Autodesk Inventor part; units mm, degrees
ref_plane "YZ Plane" through (0, 0, 0) normal (1, 0, 0) x (0, 1, 0)
ref_plane "XZ Plane" through (0, 0, 0) normal (0, 1, 0) x (-1, 0, 0)
ref_plane "XY Plane" through (0, 0, 0) normal (0, 0, 1) x (1, 0, 0)
sketch "Sketch1" plane through (0, 0, 0) normal (0, 1, 0) x (-1, 0, 0)
  line L0 (0, 0) -> (349.25, 0)
  line L1 (349.25, 0) -> (349.25, -400.05)
  line L2 (349.25, -400.05) -> (0, -400.05)
  line L3 (0, -400.05) -> (0, 0)
  dimension "d0" = 400.05
  dimension "d1" = 349.25
extrude "Extrusion1" add sketch "Sketch1" along normal blind 352.425
sketch "Sketch2" plane through (0, 0, 0) normal (1, 0, 0) x (0, 0, -1)
  line L0 (30.1625, 339.725) -> (369.8875, 339.725)
  line L1 (369.8875, 339.725) -> (369.8875, 12.7)
  line L2 (369.8875, 12.7) -> (30.1625, 12.7)
  line L3 (30.1625, 12.7) -> (30.1625, 339.725)
  line L4 (0, 0) -> (400.05, 0)
  line L5 (0, 352.425) -> (400.05, 352.425)
  line L6 (0, 0) -> (0, 352.425)
  line L7 (400.05, 0) -> (400.05, 352.425)
  dimension "d4" = 12.7
  dimension "d5" = 12.7
  dimension "d6" = 339.725
  dimension "d7" = 30.1625
  dimension "d8" = 30.1625
extrude "Extrusion2" cut sketch "Sketch2" against normal blind 333.375 contours L0 L1 L2 L3
sketch "Sketch3" plane through (0, 352.425, 0) normal (0, 1, 0) x (1, 0, 0)
  line L0 (0, 400.05) -> (-349.25, 400.05)
  line L1 (-349.25, 400.05) -> (-349.25, 0)
  line L2 (-349.25, 0) -> (0, 0)
  line L3 (0, 0) -> (0, 400.05)
extrude "Extrusion3" add sketch "Sketch3" along normal blind 174.625
sketch "Sketch4" plane through (0, 0, 0) normal (1, 0, 0) x (0, 0, -1)
  line L0 (369.8875, 339.725) -> (369.8875, 12.7)
  line L1 (369.8875, 12.7) -> (30.1625, 12.7)
  line L2 (30.1625, 12.7) -> (30.1625, 339.725)
  line L3 (30.1625, 339.725) -> (369.8875, 339.725)
  line L4 (0, 0) -> (400.05, 0)
  line L5 (400.05, 0) -> (400.05, 527.05)
  line L6 (0, 527.05) -> (400.05, 527.05)
  line L7 (0, 0) -> (0, 527.05)
  line L8 (30.1625, 501.65) -> (369.8875, 501.65)
  line L9 (369.8875, 501.65) -> (369.8875, 352.425)
  line L10 (369.8875, 352.425) -> (30.1625, 352.425)
  line L11 (30.1625, 352.425) -> (30.1625, 501.65)
  point P0 (200.025, 501.65)
  dimension "d13" = 12.7
  dimension "d14" = 25.4
extrude "Extrusion4" cut sketch "Sketch4" against normal blind 333.375 contours L8 L9 L10 L11
sketch "Sketch5" plane through (0, 527.05, 0) normal (0, 1, 0) x (1, 0, 0)
  line L0 (-349.25, 400.05) -> (-349.25, 0)
  line L1 (-349.25, 0) -> (0, 0)
  line L2 (0, 0) -> (0, 400.05)
  line L3 (0, 400.05) -> (-349.25, 400.05)
  circle A0 centre (-169.8625, 200.025) radius 63.5
  line L4 (-106.3625, 200.025) -> (0, 200.025) construction
  dimension "d17" = 127
  dimension "d20" = 106.3625
extrude "Extrusion5" cut sketch "Sketch5" against normal blind 193.675 contours A0
sketch "Sketch6" plane through (0, 527.05, 0) normal (0, 1, 0) x (1, 0, 0)
  line L0 (-312.7375, 123.825) -> (-265.1125, 123.825)
  line L1 (-265.1125, 123.825) -> (-265.1125, 276.225)
  line L2 (-265.1125, 276.225) -> (-312.7375, 276.225)
  line L3 (-312.7375, 276.225) -> (-312.7375, 123.825)
  line L4 (-349.25, 400.05) -> (-349.25, 0)
  line L5 (-349.25, 0) -> (0, 0)
  line L6 (0, 400.05) -> (-349.25, 400.05)
  line L7 (0, 0) -> (0, 400.05)
  circle A0 centre (-169.8625, 200.025) radius 63.5
  line L8 (-233.3625, 200.025) -> (-265.1125, 200.025)
  dimension "d23" = 152.4
  dimension "d24" = 47.625
  dimension "d26" = 123.825
  dimension "d27" = 123.825
  dimension "d32" = 265.1125
extrude "Extrusion6" add sketch "Sketch6" along normal blind 3.175 and the other way blind 38.1 contours L3 L2 L1 L0
properties part number "Table"
Can you work these out from the model? Positions are in its coordinate system, mm. A direction names the side the tool comes from. Give positions to 0.01 mm unless a question says otherwise; leave off trailing zeros. Loops run counter-clockwise (first coordinate to the right, second up) from the corner with the lowest first, then second, coordinate; pieces in that order, holes last. Notation, with made-up numbers: M 83.25,-11 L 129.25,-11 A11 ccw 129.25,1 Z; hole C 38,41.25 d11. An arc over 180 degrees is marked long. One line per item, written item: value. Start each with the question number.
1) Thinking about a two-plate mould opening in Z: for faces 4 (the face through (-164, 174, -30.162)), 5 (the face through (-289, 530.225, -201)), 6 (the face through (-177, 260, 0)), which applies, +Z half, -Z half, draft (parallel to the pull), parting line (faces both ways), or undercut?
2) If we section it at B-B, the plane x = -60: Give the number of separate pieces and of enclosed holes in the cut face, and give its area (3 significant figures).
3) I'm going to push flat-ended pins straight in: pin 1 (1.6 mm diameter, centred on y = 528, z = -227.5, fed in from -X); pin 2 (12 mm diameter, centred on x = -40.5, z = -179.5, fed in from +Y); pin 3 (2 mm diameter, centred on y = 312.5, z = -297, fed in from +X) (3 decimals); pin 4 (10 mm diameter, centred on x = -168.5, y = 176, fed in from +Z). Where does each tip first touch, or does it pass through?
4) If we section it at C-C, the plane z = -111.5: Write out the boundary of the cut face in (x, y) (3 decimals), and give its area (3 significant figures).
5) If I drill on line 1 (Y direction, x = -36, z = -362) (3 decimals); line 2 (Z direction, x = -209.5, y = 407); line 3 (X direction, y = 259, z = -323.5) (3 decimals), over which ranges is the centre line in solid material (lowest first)? Write a range as [from, to].
6) On a 3-axis mill with a long thin cutter (end or side, diameter ignored), from which of +Z, -Z, +X, -X, +Y, -Y can I reach the whole of each face in a straight line? I mean faces 1 (the face through (-312.738, 495, -201)), 2 (the face through (-289, 488.95, -201)), 3 (the face through (-349.25, 260, -203)). Say none if no direction works.
Completed:
1. face 4: undercut
1. face 5: draft
1. face 6: +Z half
2. separate pieces: 1
2. enclosed holes: 2
2. area: 49,100 mm^2
3. pin 1: stops at x = -312.74
3. pin 2: stops at y = 527.05
3. pin 3: stops at x = -333.375
3. pin 4: stops at z = 0
4. outline: M -349.25,0 L 0,0 L 0,12.7 L -333.375,12.7 L -333.375,339.725 L 0,339.725 L 0,352.425 L -333.375,352.425 L -333.375,501.65 L 0,501.65 L 0,527.05 L -349.25,527.05 Z
4. area: 25,300 mm^2
5. line 1: y = [0, 12.7], [339.725, 352.425], [501.65, 527.05]
5. line 2: z = [-400.05, -369.89], [-30.16, 0]
5. line 3: x = [-349.25, -333.375]
6. face 1: none
6. face 2: +X
6. face 3: +Z, -Z, -X, +Y, -Y
